Design review of the part built by this model. Coordinates are the model's own, in mm. A direction names the side the tool comes from. Round coordinates to 2 decimals unless told otherwise and drop trailing zeros. Loops run counter-clockwise (first coordinate to the right, second up) from the corner with the lowest first, then second, coordinate; pieces in that order, holes last. Notation, with made-up numbers: M -39,-9 L -24,-9 A13 cw -24,-2 Z; hole C -16,17 d8. An arc over 180 degrees is marked long. Use a Markdown table: item, result.
from build123d import *

# Parameters (mm, degrees)
F0_W      = 161
F0_H      = 21
F1_DEPTH  = 12
F2_SIZE   = 20
F3_SIZE   = 20
F5_R      = 5
F6_ANGLE  = 45
F4_R      = 5
F8_ANGLE  = 45
F9_DEPTH  = 25
F10_DEPTH = 25


with BuildPart() as f1:
    # F0 (on Top) → F1 (new body)
    with BuildSketch(Plane.XY):
        with Locations((-80.5, -10.5)):
            Rectangle(F0_W, F0_H)
    extrude(amount=F1_DEPTH)

    # F2
    f2_edges = [f1.edges().sort_by_distance(p)[0] for p in [
        (-161, 0, 6),
    ]]
    chamfer(f2_edges, length=F2_SIZE)

    # F3
    f3_edges = [f1.edges().sort_by_distance(p)[0] for p in [
        (0, 0, 6),
    ]]
    chamfer(f3_edges, length=F3_SIZE)

    # F5 (on face) → F6 (revolve)
    with BuildSketch(Plane(origin=(0, 0, 0), x_dir=(-1, 0, 0), z_dir=(0, 1, 0))):
        with Locations((132.0005953312, 5.6298593991)):
            Circle(F5_R)
    revolve(axis=Axis((-123.356834054, 0, 5.9305), (0, 0, -1)), revolution_arc=F6_ANGLE)

    # F4 (on face) → F8 (revolve)
    with BuildSketch(Plane(origin=(0, 0, 0), x_dir=(-1, 0, 0), z_dir=(0, 1, 0))):
        with Locations((29.4153820723, 5.6298593991)):
            Circle(F4_R)
    revolve(axis=Axis((-37.1628478169, 0, 5.868), (0, 0, 1)), revolution_arc=F8_ANGLE)

    # F9 (add): a face of the model
    f9_faces = [f1.faces().sort_by_distance(p)[0] for p in [
        (-129.4688962681, 6.1120622141, 5.6298593991),
    ]]
    extrude(f9_faces, amount=F9_DEPTH)

    # F10 (add): a face of the model
    f10_faces = [f1.faces().sort_by_distance(p)[0] for p in [
        (-31.6845622519, 5.478285565, 5.6298593991),
    ]]
    extrude(f10_faces, amount=F10_DEPTH)


solid = f1.part
1. Take a section at B-B on y = -10.5. Give the boundary of the cut face in (x, z).
Check values:
| item | result |
|---|---|
| outline | M -151.5,0 L -9.5,0 L -9.5,12 L -151.5,12 Z |
2. The part is to be moulded in two halves that separate along Y. For faces 3 (the face through (-82, -21, 6)), 4 (the face through (-43.77, 10.82, 7.13)), 5 (the face through (-112, 24, 6)), say which applies: pulls with the +Y half, pulls with the -Y half, needs draft (parallel to the pull), parting line crosses it, or undercut.
Check values:
| item | result |
|---|---|
| face 3 | pulls with the -Y half |
| face 4 | undercut |
| face 5 | pulls with the +Y half |
3. Insertion check: pin 1 (3 mm diameter, centred on x = -88, z = 8.5, fed in from +Y); pin 2 (1.5 mm diameter, centred on x = -38.5, y = 9, fed in from +Z); pin 3 (3 mm diameter, centred on y = -2.5, z = 8, fed in from +X). Each pin has a flat end and moves straight along its axis. Give the tip position at first contact, or say it passes through.
Check values:
| item | result |
|---|---|
| pin 1 | stops at y = 0 |
| pin 2 | stops at z = 10.37 |
| pin 3 | stops at x = -16 |
4. Machinability: for faces 1 (the face through (-49.31, 23.21, 5.7)), 2 (the face through (-10, -10, 6)), which of the approach directions +Z, -Z, +X, -X, +Y, -Y give a long, thin tool a straight path to every point of the face, cutting with its end or side? Answer none if there is none.
Check values:
| item | result |
|---|---|
| face 1 | +Z, -Z, +Y |
| face 2 | +Z, -Z, +X, +Y |
5. Take a section at C-C on x = -84.5. Give the boundary of the cut face in (y, z), and give its area (3 significant figures).
Check values:
| item | result |
|---|---|
| outline | M -21,0 L 0,0 L 0,12 L -21,12 Z |
| area | 252 mm² |
6. Take a section at A-A on z = 3. Give the boundary of the cut face in (x, y), and give its area (3 significant figures).
Check values:
| item | result |
|---|---|
| outline | M -161,-21 L 0,-21 L 0,-20 L -20,0 L -25.16,0 A12 ccw -28.68,8.49 L -46.36,26.16 L -52.37,20.15 L -34.69,2.47 A3.49 cw -33.67,0 L -127.75,0 A4.39 cw -126.46,3.11 L -108.78,20.78 L -114.8,26.8 L -132.48,9.12 A12.9 ccw -136.25,0 L -141,0 L -161,-20 Z |
| area | 3,520 mm² |
7. Wall thickness on line 1 along Y through (x, z) = (-118, 1.75); line 2 along Y through (x, z) = (-64, 1); line 3 along X through (y, z) = (25, 5.25): over which ranges is each line inside the solid? List them lowest first. Write a range as from..to.
Check values:
| item | result |
|---|---|
| line 1 | y = -21..0, 13.12..22.04 |
| line 2 | y = -21..0 |
| line 3 | x = -117.63..-113, -47.52..-44.16 |
